The listing builds one solid part. Answer for the finished solid, in the listing's coordinates (mm). A direction names the side the tool comes from. Coordinates: 2 decimals unless noted, no trailing zeros. Order: outer loops, then holes, each group sorted by start corner. A loop starts at its lowest first (then second) coordinate and runs counter-clockwise, first axis right, second up. Notation, with made-up numbers: (1, 70) -> (30, 70) arc R23 ccw to (30, 108) -> close; hole circle Ø3 at (23.25, 41). An arc over 180 degrees is marked (long way). Return JSON: item names as keys, results as strings.
```python
from build123d import *

# Parameters (mm, degrees)
SKETCH_5_W          = 55
SKETCH_5_H          = 3
EXTRUDE_1_DEPTH     = 5
CUT_EXTRUDE_1_REACH = 57.308
SKETCH_6_R          = 1.6
CUT_EXTRUDE_2_REACH = 57.308
SKETCH_7_R          = 0.9
FILLET_1_R          = 1.5
SKETCH_8_W          = 6
SKETCH_8_H          = 1.6
CUT_EXTRUDE_3_DEPTH = 10
SKETCH_10_R         = 1.6
SKETCH_10_R_2       = 0.9
EXTRUDE_2_DEPTH     = 0.5
EXTRUDE_START       = 0.5
SKETCH_11_R         = 0.9
SKETCH_11_R_2       = 1.6
EXTRUDE_3_DEPTH     = 0.5
SKETCH_12_W         = 6.953496512
SKETCH_12_H         = 2
CUT_EXTRUDE_4_DEPTH = 10


with BuildPart() as part:
    # 草图5 → 凸台-拉伸1 (new body)
    with BuildSketch(Plane(origin=(0, 0, 0), x_dir=(1, 0, 0), z_dir=(0, 1, 0))):
        with Locations((27.5, -1.5)):
            Rectangle(SKETCH_5_W, SKETCH_5_H)
    extrude(amount=EXTRUDE_1_DEPTH)

    # 草图6 → 切除-拉伸1 (cut, up to next)
    with BuildSketch(Plane.XY.offset(3), mode=Mode.PRIVATE) as cut_extrude_1_sk1:
        with Locations((2.5, 2.5)):
            Circle(SKETCH_6_R)
    cut_extrude_1_tool1 = extrude(cut_extrude_1_sk1.sketch, amount=-CUT_EXTRUDE_1_REACH, mode=Mode.PRIVATE) & part.part
    add(cut_extrude_1_tool1.solids().sort_by_distance((2.5, 2.5, 3))[0], mode=Mode.SUBTRACT)

    # 草图7 → 切除-拉伸2 (cut, up to next)
    with BuildSketch(Plane.XY, mode=Mode.PRIVATE) as cut_extrude_2_sk1:
        with Locations(Location((53, 2.5, 0), (0, 0, 180))):
            Circle(SKETCH_7_R)
    cut_extrude_2_tool1 = extrude(cut_extrude_2_sk1.sketch, amount=CUT_EXTRUDE_2_REACH, mode=Mode.PRIVATE) & part.part
    add(cut_extrude_2_tool1.solids().sort_by_distance((53, 2.5, 0))[0], mode=Mode.SUBTRACT)

    # 圆角1
    fillet_1_edges = [part.edges().sort_by_distance(p)[0] for p in [
        (55, 5, 1.5),
        (55, 0, 1.5),
        (0, 0, 1.5),
        (0, 5, 1.5),
    ]]
    fillet(fillet_1_edges, radius=FILLET_1_R)

    # 草图8 → 切除-拉伸3 (cut)
    with BuildSketch(Plane(origin=(0, 5, 0), x_dir=(1, 0, 0), z_dir=(0, 1, 0))):
        with Locations((52, -1.5)):
            Rectangle(SKETCH_8_W, SKETCH_8_H)
    extrude(amount=-CUT_EXTRUDE_3_DEPTH, mode=Mode.SUBTRACT)

    # 草图10 → 凸台-拉伸2 (add)
    with BuildSketch(Plane.XY.offset(3)):
        with BuildLine():
            Line((0, 3.5), (0, 1.5))
            ThreePointArc((0, 1.5), (0.439339828, 0.439339828), (1.5, 0))
            Line((1.5, 0), (53.5, 0))
            ThreePointArc((53.5, 0), (54.560660172, 0.439339828), (55, 1.5))
            Line((55, 1.5), (55, 3.5))
            ThreePointArc((55, 3.5), (54.560660172, 4.560660172), (53.5, 5))
            Line((53.5, 5), (1.5, 5))
            ThreePointArc((1.5, 5), (0.439339828, 4.560660172), (0, 3.5))
        make_face()
        with Locations((2.5, 2.5)):
            Circle(SKETCH_10_R, mode=Mode.SUBTRACT)
        with Locations((53, 2.5)):
            Circle(SKETCH_10_R_2, mode=Mode.SUBTRACT)
    extrude(amount=EXTRUDE_2_DEPTH)

    # 草图11 → 凸台-拉伸3 (add)
    with BuildSketch(Plane(origin=(0, 0, 0), x_dir=(-1, 0, 0), z_dir=(0, 0, -1)).offset(EXTRUDE_START)):
        with BuildLine():
            Line((-1.5, 5), (-53.5, 5))
            ThreePointArc((-53.5, 5), (-54.560660172, 4.560660172), (-55, 3.5))
            Line((-55, 3.5), (-55, 1.5))
            ThreePointArc((-55, 1.5), (-54.560660172, 0.439339828), (-53.5, 0))
            Line((-53.5, 0), (-1.5, 0))
            ThreePointArc((-1.5, 0), (-0.439339828, 0.439339828), (0, 1.5))
            Line((0, 1.5), (0, 3.5))
            ThreePointArc((0, 3.5), (-0.439339828, 4.560660172), (-1.5, 5))
        make_face()
        with Locations(Location((-53, 2.5, 0), (0, 0, 180))):
            Circle(SKETCH_11_R, mode=Mode.SUBTRACT)
        with Locations(Location((-2.5, 2.5, 0), (0, 0, 180))):
            Circle(SKETCH_11_R_2, mode=Mode.SUBTRACT)
    extrude(amount=-EXTRUDE_3_DEPTH)

    # 草图12 → 切除-拉伸4 (cut)
    with BuildSketch(Plane(origin=(0, 5, 0), x_dir=(1, 0, 0), z_dir=(0, 1, 0))):
        with Locations((52.476748256, -1.5)):
            Rectangle(SKETCH_12_W, SKETCH_12_H)
    extrude(amount=-CUT_EXTRUDE_4_DEPTH, mode=Mode.SUBTRACT)


solid = part.part
```
Item 1: Determine the mould class of faces 3 (the flat face through (28, 3, -0.5)), 4 (the flat face through (49, 3, 2)), 5 (the flat face through (27, 5, 1)), 6 (the flat face through (27, 3, 3.5)) for opening direction Z: pulls with the +Z half, pulls with the -Z half, needs draft (parallel to the pull), parting line crosses it, or undercut.
Answer list:
{"face 3": "pulls with the -Z half", "face 4": "undercut", "face 5": "needs draft", "face 6": "pulls with the +Z half"}
Item 2: The part is cut by section D-D on x = 53. Determine the outline of the cut face in (y, z), plus the area to 3 significant figures.
Answer list:
{"outline": "(0, -0.5) -> (1.6, -0.5) -> (1.6, 0.5) -> (0, 0.5) -> close; (0, 2.5) -> (1.6, 2.5) -> (1.6, 3.5) -> (0, 3.5) -> close; (3.4, -0.5) -> (5, -0.5) -> (5, 0.5) -> (3.4, 0.5) -> close; (3.4, 2.5) -> (5, 2.5) -> (5, 3.5) -> (3.4, 3.5) -> close", "area": "6.40 mm2"}
Item 3: The part is cut by section B-B on x = 2.5. Determine the outline of the cut face in (y, z), plus the area to 3 significant figures.
Answer list:
{"outline": "(0, -0.5) -> (0.9, -0.5) -> (0.9, 3.5) -> (0, 3.5) -> close; (4.1, -0.5) -> (5, -0.5) -> (5, 3.5) -> (4.1, 3.5) -> close", "area": "7.20 mm2"}
Item 4: The part is cut by section C-C on z = 2.05. Determine the outline of the cut face in (x, y).
Answer list:
{"outline": "(0, 1.5) arc R1.5 ccw to (1.5, 0) -> (49, 0) -> (49, 5) -> (1.5, 5) arc R1.5 ccw to (0, 3.5) -> close; hole circle Ø3.2 at (2.5, 2.5)"}
Item 5: The part is cut by section A-A on y = 2.5. Determine the outline of the cut face in (x, z), plus the area to 3 significant figures.
Answer list:
{"outline": "(0, -0.5) -> (0.9, -0.5) -> (0.9, 3.5) -> (0, 3.5) -> close; (4.1, -0.5) -> (52.1, -0.5) -> (52.1, 0.5) -> (49, 0.5) -> (49, 2.5) -> (52.1, 2.5) -> (52.1, 3.5) -> (4.1, 3.5) -> close; (53.9, -0.5) -> (55, -0.5) -> (55, 0.5) -> (53.9, 0.5) -> close; (53.9, 2.5) -> (55, 2.5) -> (55, 3.5) -> (53.9, 3.5) -> close", "area": "192 mm2"}
Item 6: Which of the six approach directions +Z, -Z, +X, -X, +Y, -Y give full straight-line access (tool end or side, diameter ignored) to faces 1 (the cylindrical face through (0.43, 4.55, 1.47)), 2 (the flat face through (52, 3, 0.5))?
Answer list:
{"face 1": "+Z, -Z, -X, +Y", "face 2": "+X, +Y, -Y"}
Item 7: A flat-ended cylindrical pin translates along its axis: pin 1 (2.5 mm diameter, centred on x = 2.5, y = 2.5, fed in from +Z). Find the tip coordinate at first contact, or state that the pin passes through.
Answer list:
{"pin 1": "through"}
Item 8: Find the intervals of material crossed by probe 1 along Z at (x, y) = (51.5, 4.6); probe 2 along X at (y, z) = (2.5, -0.3); probe 3 along Y at (x, z) = (2.5, -0.15), in increasing order.
Answer list:
{"probe 1": "-0.5 to 0.5, 2.5 to 3.5", "probe 2": "0 to 0.9, 4.1 to 52.1, 53.9 to 55", "probe 3": "0 to 0.9, 4.1 to 5"}
